```python
from build123d import *

# Parameters (mm, degrees)
SKETCH1_W            = 160
SKETCH1_H            = 160
BOSS_EXTRUDE1_DEPTH  = 5
BOSS_EXTRUDE8_DEPTH  = 35
BOSS_EXTRUDE11_DEPTH = 80
SKETCH23_W           = 160
SKETCH23_H           = 10
BOSS_EXTRUDE12_DEPTH = 20
SKETCH25_W           = 21.5
SKETCH25_H           = 180
CUT_EXTRUDE4_DEPTH   = 10


with BuildPart() as part:
    # Sketch1 → Boss-Extrude1 (new, symmetric)
    with BuildSketch(Plane(origin=(0, 0, 0), x_dir=(1, 0, 0), z_dir=(0, 1, 0))):
        Rectangle(SKETCH1_W, SKETCH1_H)
    extrude(amount=BOSS_EXTRUDE1_DEPTH, both=True)

    # Sketch17 → Boss-Extrude8 (add)
    with BuildSketch(Plane(origin=(0, 5, 0), x_dir=(1, 0, 0), z_dir=(0, 1, 0))):
        with BuildLine():
            Line((-6.135166846, 3.859212979), (-6.135166846, -1.338646794))
            ThreePointArc((-6.135166846, -1.338646794), (0, 48.1), (6.135166846, -1.338646794))
            Line((6.135166846, -1.338646794), (6.135166846, 3.859212979))
            ThreePointArc((6.135166846, 3.859212979), (0, 43.1), (-6.135166846, 3.859212979))
        make_face()
    extrude(amount=BOSS_EXTRUDE8_DEPTH)

    # Sketch19 → Boss-Extrude11 (add)
    with BuildSketch(Plane(origin=(0, 5, 0), x_dir=(1, 0, 0), z_dir=(0, 1, 0))):
        Polygon((-80, 80), (-80, -30.581038256), (-70, -30.581038256), (-70, 70), (48.5, 70), (48.5, 25.826966248), (48.5, -30.581038256), (58.5, -30.581038256), (58.5, 25.826966248), (58.5, 74), (58.5, 80), (-70, 80), align=None)
    extrude(amount=BOSS_EXTRUDE11_DEPTH)

    # Sketch23 → Boss-Extrude12 (add)
    with BuildSketch(Plane(origin=(0, 0, -80), x_dir=(-1, 0, 0), z_dir=(0, 0, -1))):
        Rectangle(SKETCH23_W, SKETCH23_H)
    extrude(amount=BOSS_EXTRUDE12_DEPTH)

    # Sketch25 → Cut-Extrude4 (cut)
    with BuildSketch(Plane(origin=(0, 5, 0), x_dir=(1, 0, 0), z_dir=(0, 1, 0))):
        with Locations((69.25, 10)):
            Rectangle(SKETCH25_W, SKETCH25_H)
    extrude(amount=-CUT_EXTRUDE4_DEPTH, mode=Mode.SUBTRACT)


solid = part.part
```
Source: CAD feature listing. Evaluate the final solid. Frame: model axes, mm. A direction names the side the tool comes from. Round coordinates to 2 decimals unless told otherwise and drop trailing zeros. Order: outer loops, then holes, each group sorted by start corner. A loop starts at its lowest first (then second) coordinate and runs counter-clockwise, first axis right, second up. Notation, with made-up numbers: (-19.5, -26.75) -> (16.5, -26.75) arc R20 cw to (16.5, -1.75) -> close; hole circle Ø7 at (-28.5, 79.25). An arc over 180 degrees is marked (long way). Use CSV: the item, a comma, the result in double quotes.
(1) Ray query, L1, parallel to X at y = 16, z = -23; L2, parallel to X at y = 30, z = -64.5; L3, parallel to Z at x = 0, y = 20. Return the intervals inside material, ascending.
Report:
L1,"-80 to -70, -25.1 to -20.1, 20.1 to 25.1, 48.5 to 58.5"
L2,"-80 to -70, 48.5 to 58.5"
L3,"-80 to -70, -48.1 to -43.1"
(2) Access query for faces 5 (the face through (53, 44, 30.581)), 6 (the face through (-70, 44, -19)), 7 (the face through (-12, 44, -70)). Directions: +Z, -Z, +X, -X, +Y, -Y. A direction counts if a zero-diameter tool reaches every point of the face in a straight line with its end or side. Return the directions, or none.
Report:
face 5,"+Z, +X, -X, +Y"
face 6,"+Z, +Y"
face 7,"+Y"
(3) First-contact query: pin 1 Ø6 at (x, z) = (-37.5, -90.5) entering from +Y; pin 2 Ø4 at (x, y) = (1.5, 33) entering from +Z; pin 3 Ø12 at (x, y) = (5.5, 58) entering from +Z. Flat tips, straight axial feed; report the tip coordinate or a pass-through.
Report:
pin 1,"y = 5"
pin 2,"z = -42.79"
pin 3,"z = -70"
(4) Section C-C on x = 0. Return the cut outline in (y, z).
Report:
outline,"(-5, -100) -> (5, -100) -> (5, -80) -> (85, -80) -> (85, -70) -> (5, -70) -> (5, -48.1) -> (40, -48.1) -> (40, -43.1) -> (5, -43.1) -> (5, 80) -> (-5, 80) -> close"
(5) Section B-B on z = -23. Return the cut outline in (x, y).
Report:
outline,"(-80, -5) -> (58.5, -5) -> (58.5, 85) -> (48.5, 85) -> (48.5, 5) -> (25.1, 5) -> (25.1, 40) -> (20.1, 40) -> (20.1, 5) -> (-20.1, 5) -> (-20.1, 40) -> (-25.1, 40) -> (-25.1, 5) -> (-70, 5) -> (-70, 85) -> (-80, 85) -> close"
(6) Section D-D on y = 78. Return the cut outline in (x, z).
Report:
outline,"(-80, -80) -> (58.5, -80) -> (58.5, 30.58) -> (48.5, 30.58) -> (48.5, -70) -> (-70, -70) -> (-70, 30.58) -> (-80, 30.58) -> close"
(7) Section A-A on y = 22.5. Return the cut outline in (x, z).
Report:
outline,"(-80, -80) -> (58.5, -80) -> (58.5, 30.58) -> (48.5, 30.58) -> (48.5, -70) -> (-70, -70) -> (-70, 30.58) -> (-80, 30.58) -> close; (-6.14, -3.86) -> (-6.14, 1.34) arc R25.1 ccw (long way) to (6.14, 1.34) -> (6.14, -3.86) arc R20.1 cw (long way) to start"
(8) Pull-direction query (Z, two-part tool) for faces 1 (the face through (-1.02, 22.26, -48.08)), 2 (the face through (6.135, 22, -1)), 3 (the face through (-10, 44, -80)), 4 (the face through (-75, 44, 30.581)); classes: +Z half, -Z half, draft (parallel to the pull), parting line (faces both ways), or undercut.
Report:
face 1,"undercut"
face 2,"draft"
face 3,"-Z half"
face 4,"+Z half"
